from build123d import *

# Parameters (mm, degrees)
SKETCH_1_W          = 40
SKETCH_1_H          = 20
SKETCH_1_W_2        = 38
SKETCH_1_H_2        = 18
EXTRUDE_1_DEPTH     = 150
SKETCH_2_R          = 6.55
CUT_EXTRUDE_1_DEPTH = 40
SKETCH_3_R          = 1.55
CUT_EXTRUDE_2_DEPTH = 30
SKETCH_4_R          = 4
CUT_EXTRUDE_3_DEPTH = 10
SKETCH_5_R          = 1.6
CUT_EXTRUDE_4_DEPTH = 50
SKETCH_6_R          = 1.6
SKETCH_6_R_2        = 2.1
CUT_EXTRUDE_5_DEPTH = 50
SKETCH_7_R          = 10
SKETCH_7_R_2        = 1.55
CUT_EXTRUDE_6_DEPTH = 30
SKETCH_10_R         = 6
CUT_EXTRUDE_7_DEPTH = 50


with BuildPart() as part:
    # 草图1 → 凸台-拉伸1 (new, symmetric)
    with BuildSketch(Plane.XY):
        Rectangle(SKETCH_1_W, SKETCH_1_H)
        Rectangle(SKETCH_1_W_2, SKETCH_1_H_2, mode=Mode.SUBTRACT)
    extrude(amount=EXTRUDE_1_DEPTH, both=True)

    # 草图2 → 切除-拉伸1 (cut)
    with BuildSketch(Plane(origin=(20, 0, 0), x_dir=(0, 0, -1), z_dir=(1, 0, 0))):
        with Locations((-140, 0)):
            Circle(SKETCH_2_R)
        with Locations((140, 0)):
            Circle(SKETCH_2_R)
    extrude(amount=-CUT_EXTRUDE_1_DEPTH, mode=Mode.SUBTRACT)

    # 草图3 → 切除-拉伸2 (cut)
    with BuildSketch(Plane(origin=(0, 10, 0), x_dir=(1, 0, 0), z_dir=(0, 1, 0))):
        with Locations(Location((-14, -84, 0), (0, 0, 270))):
            Circle(SKETCH_3_R)
        with Locations(Location((-14, -66, 0), (0, 0, 270))):
            Circle(SKETCH_3_R)
        with Locations(Location((14, -84, 0), (0, 0, 270))):
            Circle(SKETCH_3_R)
        with Locations(Location((14, -66, 0), (0, 0, 270))):
            Circle(SKETCH_3_R)
        with Locations(Location((-14, 66, 0), (0, 0, 270))):
            Circle(SKETCH_3_R)
        with Locations(Location((-14, 84, 0), (0, 0, 270))):
            Circle(SKETCH_3_R)
        with Locations(Location((14, 66, 0), (0, 0, 270))):
            Circle(SKETCH_3_R)
        with Locations(Location((14, 84, 0), (0, 0, 270))):
            Circle(SKETCH_3_R)
    extrude(amount=-CUT_EXTRUDE_2_DEPTH, mode=Mode.SUBTRACT)

    # 草图4 → 切除-拉伸3 (cut)
    with BuildSketch(Plane.XZ.offset(10)):
        with Locations(Location((14, -84, 0), (0, 0, 270))):
            Circle(SKETCH_4_R)
        with Locations(Location((14, -66, 0), (0, 0, 270))):
            Circle(SKETCH_4_R)
        with Locations(Location((14, 84, 0), (0, 0, 270))):
            Circle(SKETCH_4_R)
        with Locations(Location((14, 66, 0), (0, 0, 270))):
            Circle(SKETCH_4_R)
    extrude(amount=-CUT_EXTRUDE_3_DEPTH, mode=Mode.SUBTRACT)

    # 草图5 → 切除-拉伸4 (cut)
    with BuildSketch(Plane(origin=(20, 0, 0), x_dir=(0, 0, -1), z_dir=(1, 0, 0))):
        with Locations((122, 5)):
            Circle(SKETCH_5_R)
        with Locations((122, -5)):
            Circle(SKETCH_5_R)
        with Locations((107, 5)):
            Circle(SKETCH_5_R)
        with Locations((107, -5)):
            Circle(SKETCH_5_R)
        with Locations((-107, -5)):
            Circle(SKETCH_5_R)
        with Locations((-107, 5)):
            Circle(SKETCH_5_R)
        with Locations((-122, -5)):
            Circle(SKETCH_5_R)
        with Locations((-122, 5)):
            Circle(SKETCH_5_R)
    extrude(amount=-CUT_EXTRUDE_4_DEPTH, mode=Mode.SUBTRACT)

    # 草图6 → 切除-拉伸5 (cut)
    with BuildSketch(Plane.XZ.offset(10)):
        with Locations(Location((-14.5, -130.5, 0), (0, 0, 270))):
            Circle(SKETCH_6_R)
        with Locations(Location((14.5, -130.5, 0), (0, 0, 270))):
            Circle(SKETCH_6_R)
        with Locations(Location((14.5, -112, 0), (0, 0, 270))):
            Circle(SKETCH_6_R_2)
        with Locations(Location((-14.5, -112, 0), (0, 0, 270))):
            Circle(SKETCH_6_R_2)
        with Locations(Location((-14.5, 112, 0), (0, 0, 90))):
            Circle(SKETCH_6_R_2)
        with Locations(Location((14.5, 112, 0), (0, 0, 90))):
            Circle(SKETCH_6_R_2)
        with Locations(Location((14.5, 130.5, 0), (0, 0, 90))):
            Circle(SKETCH_6_R)
        with Locations(Location((-14.5, 130.5, 0), (0, 0, 90))):
            Circle(SKETCH_6_R)
    extrude(amount=-CUT_EXTRUDE_5_DEPTH, mode=Mode.SUBTRACT)

    # 草图7 → 切除-拉伸6 (cut)
    with BuildSketch(Plane(origin=(0, 10, 0), x_dir=(1, 0, 0), z_dir=(0, 1, 0))):
        with Locations(Location((0, 30, 0), (0, 0, 270))):
            Circle(SKETCH_7_R)
        with Locations(Location((14, 44, 0), (0, 0, 270))):
            Circle(SKETCH_7_R_2)
        with Locations(Location((-14, 44, 0), (0, 0, 270))):
            Circle(SKETCH_7_R_2)
        with Locations(Location((-14, 16, 0), (0, 0, 270))):
            Circle(SKETCH_7_R_2)
        with Locations(Location((14, 16, 0), (0, 0, 270))):
            Circle(SKETCH_7_R_2)
        with Locations(Location((14, -16, 0), (0, 0, 270))):
            Circle(SKETCH_7_R_2)
        with Locations(Location((-14, -16, 0), (0, 0, 270))):
            Circle(SKETCH_7_R_2)
        with Locations(Location((-14, -44, 0), (0, 0, 270))):
            Circle(SKETCH_7_R_2)
        with Locations(Location((14, -44, 0), (0, 0, 270))):
            Circle(SKETCH_7_R_2)
        with Locations(Location((0, -30, 0), (0, 0, 270))):
            Circle(SKETCH_7_R)
    extrude(amount=-CUT_EXTRUDE_6_DEPTH, mode=Mode.SUBTRACT)

    # 草图10 → 切除-拉伸7 (cut)
    with BuildSketch(Plane(origin=(20, 0, 0), x_dir=(0, 0, -1), z_dir=(1, 0, 0))):
        with Locations((55, 0)):
            Circle(SKETCH_10_R)
        with Locations((-55, 0)):
            Circle(SKETCH_10_R)
        with BuildLine():
            Line((-7.5, 5), (7.5, 5))
            ThreePointArc((7.5, 5), (12.5, 0), (7.5, -5))
            Line((7.5, -5), (-7.5, -5))
            ThreePointArc((-7.5, -5), (-12.5, 0), (-7.5, 5))
        make_face()
    extrude(amount=-CUT_EXTRUDE_7_DEPTH, mode=Mode.SUBTRACT)


solid = part.part
Read the model definition and answer for the solid it produces. Units are mm, in the model's axes. A direction names the side the tool comes from. Round coordinates to 2 decimals unless told otherwise and drop trailing zeros. Order: outer loops, then holes, each group sorted by start corner. A loop starts at its lowest first (then second) coordinate and runs counter-clockwise, first axis right, second up. Notation, with made-up numbers: (37, 35.25) - (64, 35.25) arc R30 cw to (64, 68.25) - close; hole circle Ø9 at (52, 76.25). An arc over 180 degrees is marked (long way). Use one line per item in the form item = value. Start each with the question number.
(1) Find the intervals of material crossed by line 1 along X through (y, z) = (9.75, 44); line 2 along X through (y, z) = (9.4, -112); line 3 along Y through (x, z) = (19.45, 107), in increasing order. Write a range as from..to.
(2) For faces 4 (the face through (-19, -6, 2)), 5 (the face through (-19.5, -0.1, 12.5)), 6 (the face through (15.201, -9.507, -69.815)), determine the directions among +Z, -Z, +X, -X, +Y, -Y from which every point of the face is accessible in a straight line to the end or side of a thin tool.
(3) The part is cut by section A-A (z = 4.5). Give the vertices of the cut face in (x, y), then the cut area to 3 significant figures.
(4) The part is cut by section B-B (x = 0). Give the vertices of the cut face in (y, z).
(5) Flat-ended cylindrical pins translate along their axes: pin 1 Ø2.5 at (x, z) = (14, 66) entering from -Y; pin 2 Ø4 at (x, z) = (14, -84) entering from -Y; pin 3 Ø8 at (x, z) = (6, 37) entering from -Y. Find the tip coordinate at first contact, or state that the pin passes through.
(6) The part is cut by section C-C (z = -30). Give the vertices of the cut face in (x, y).
(7) Determine the mould class of faces 1 (the face through (-20, 7, 2)), 2 (the face through (0, -9, 2)), 3 (the face through (-19.493, 0.264, -49.006)) for opening direction X: +X half, -X half, draft (parallel to the pull), parting line (faces both ways), or undercut.
(8) The part is cut by section D-D (y = 0). Count the separate pieces of the cut face and the enclosed holes in it, then the cut area to 3 significant figures.
Checked values:
q1.line_1 = -20..-15.55, -12.45..12.45, 15.55..20
q1.line_2 = -20..-16.6, -12.4..12.4, 16.6..20
q1.line_3 = -10..-6.6, -3.4..3.4, 6.6..10
q2.face_4 = +Z, -Z
q2.face_5 = +X, -X
q2.face_6 = -Y
q3.outline = (-20, -10) - (20, -10) - (20, -5) - (19, -5) - (19, -9) - (-19, -9) - (-19, -5) - (-20, -5) - close; (-20, 5) - (-19, 5) - (-19, 9) - (19, 9) - (19, 5) - (20, 5) - (20, 10) - (-20, 10) - close
q3.area = 96.0 mm^2
q4.outline = (-10, -150) - (-9, -150) - (-9, -40) - (-10, -40) - close; (-10, -20) - (-9, -20) - (-9, 20) - (-10, 20) - close; (-10, 40) - (-9, 40) - (-9, 150) - (-10, 150) - close; (9, -150) - (10, -150) - (10, -40) - (9, -40) - close; (9, -20) - (10, -20) - (10, 20) - (9, 20) - close; (9, 40) - (10, 40) - (10, 150) - (9, 150) - close
q5.pin_1 = through
q5.pin_2 = 9
q5.pin_3 = -10
q6.outline = (-20, -10) - (-10, -10) - (-10, -9) - (-19, -9) - (-19, 9) - (-10, 9) - (-10, 10) - (-20, 10) - close; (10, -10) - (20, -10) - (20, 10) - (10, 10) - (10, 9) - (19, 9) - (19, -9) - (10, -9) - close
q7.face_1 = -X half
q7.face_2 = undercut
q7.face_3 = draft
q8.separate_pieces = 12
q8.enclosed_holes = 0
q8.area = 450 mm^2
